Can you work these out from the model? Positions are in its coordinate system, mm. A direction names the side the tool comes from. Round coordinates to 2 decimals unless told otherwise and drop trailing zeros. Write each loop counter-clockwise with the first axis right and the second up, starting at its lowest first coordinate (ties: lowest second). Pieces come first, ordered by that corner, then holes. Notation, with made-up numbers: M -10.5,26 L 48.5,26 A9 cw 48.5,31 Z; hole C 86.25,30.25 d8. An arc over 180 degrees is marked long. Answer as a JSON object with one key per item and string values. Group by question number.
1) Please list where these lines run through material, in increasing order: L1, parallel to X at y = 5.25, z = 2.2; L2, parallel to Z at x = 17.25, y = 7; L3, parallel to Y at x = -2, z = 0.6. Write a range as [from, to].
2) Suppose I cut it at D-D, the plane y = 2.5. Write out the boundary of the cut face in (x, z), and give its area (3 significant figures).
3) Suppose I cut it at C-C, the plane x = 17.25. Write out the boundary of the cut face in (y, z), and give its area (3 significant figures).
4) If we mould it in two halves opening along Y, with no side actions, what happens to faces 5 (the flat face through (10, 3.051, 2)), 6 (the flat face through (7, 8, 0)), 7 (the cylindrical face through (-5.414, 8.228, 0.811)), 8 (the cylindrical face through (-2.325, 7.536, 0.811))? For each: +Y half, -Y half, draft (parallel to the pull), parting line (faces both ways), or undercut.
5) I'm going to push flat-ended pins straight in: pin 1 Ø1.5 at (x, z) = (10, 2.5) entering from -Y; pin 2 Ø1.1 at (y, z) = (6, 2.5) entering from -X; pin 3 Ø0.5 at (y, z) = (2.5, 0.5) entering from +X. Where does each tip first touch, or does it pass through?
6) Suppose I cut it at A-A, the plane z = 0.7. Write out the boundary of the cut face in (x, y).
7) Suppose I cut it at B-B, the plane y = 9. Write out the boundary of the cut face in (x, z).
8) On a 3-axis mill with a long thin cutter (end or side, diameter ignored), from which of +Z, -Z, +X, -X, +Y, -Y can I reach the whole of each face in a straight line? I mean faces 1 (the flat face through (4, 8.379, 2)), 2 (the flat face through (2.571, 7, 2)), 3 (the flat face through (15, 2, 1)), 4 (the flat face through (10, 7.068, 2)). Say none if no direction works.
from build123d import *

# Parameters (mm, degrees)
SKETCH_1_W      = 15
SKETCH_1_H      = 13
EXTRUDE_1_DEPTH = 1.6
SKETCH_2_R      = 3.5
SKETCH_2_R_2    = 1.5
EXTRUDE_2_DEPTH = 1.6
FILLET_1_R      = 2
SKETCH_3_W      = 3.618558991
SKETCH_3_H      = 4.017455257
SKETCH_3_W_2    = 2.3933776
SKETCH_3_H_2    = 3.647051581
EXTRUDE_3_DEPTH = 1.4
EXTRUDE_4_DEPTH = 1.6


with BuildPart() as part:
    # Эскиз1 → Бобышка-Вытянуть1 (new body)
    with BuildSketch(Plane.XY):
        with Locations((7.5, 6.5)):
            Rectangle(SKETCH_1_W, SKETCH_1_H)
    extrude(amount=EXTRUDE_1_DEPTH)

    # Эскиз2 → Бобышка-Вытянуть2 (add)
    # profile 1 of 2: a face of its own
    with BuildSketch(Plane.XY.offset(1.6)):
        with Locations((-2, 9)):
            Circle(SKETCH_2_R)
        with Locations((-2, 9)):
            Circle(SKETCH_2_R_2, mode=Mode.SUBTRACT)
    # profile 2 of 2: a face of its own
    with BuildSketch(Plane.XY.offset(1.6)):
        with Locations((17, 9)):
            Circle(SKETCH_2_R)
        with Locations(Location((17, 9, 0), (0, 0, 180))):
            Circle(SKETCH_2_R_2, mode=Mode.SUBTRACT)
    extrude(amount=-EXTRUDE_2_DEPTH)

    # Скругление1
    fillet_1_edges = [part.edges().sort_by_distance(p)[0] for p in [
        (0, 6.127718677, 0.8),
        (15, 6.127718677, 0.8),
    ]]
    fillet(fillet_1_edges, radius=FILLET_1_R)

    # Эскиз3 → Бобышка-Вытянуть3 (add)
    with BuildSketch(Plane.XY.offset(1.6)):
        with Locations((9.793653534, 5.059744515)):
            Rectangle(SKETCH_3_W, SKETCH_3_H)
        with Locations((3.767470648, 6.555605515)):
            Rectangle(SKETCH_3_W_2, SKETCH_3_H_2)
    extrude(amount=EXTRUDE_3_DEPTH)

    # Эскиз4 → Бобышка-Вытянуть4 (add)
    with BuildSketch(Plane.XY.offset(1.6)):
        with BuildLine():
            Line((-3.62195122, 12.101495485), (7.5, 9.632875059))
            Line((7.5, 9.632875059), (18.62195122, 12.101495485))
            ThreePointArc((18.62195122, 12.101495485), (7.5, 14.834097875), (-3.62195122, 12.101495485))
        make_face()
    extrude(amount=-EXTRUDE_4_DEPTH)


solid = part.part
Results:
{
 "1": {"L1": "[2.57, 4.96], [7.98, 11.6]", "L2": "[0, 1.6]", "L3": "[5.5, 7.5], [10.5, 12.87]"},
 "2": {"outline": "M 0,0 L 15,0 L 15,1.6 L 0,1.6 Z", "area": "24.0 mm^2"},
 "3": {"outline": "M 5.51,0 L 7.52,0 L 7.52,1.6 L 5.51,1.6 Z; M 10.48,0 L 12.76,0 L 12.76,1.6 L 10.48,1.6 Z", "area": "6.88 mm^2"},
 "4": {"face 5": "-Y half", "face 6": "draft", "face 7": "parting line", "face 8": "undercut"},
 "5": {"pin 1": "y = 3.05", "pin 2": "x = 2.57", "pin 3": "x = 15"},
 "6": {"outline": "M -3.62,12.1 A3.5 ccw -2,5.5 A2 cw 0,3.5 L 0,0 L 15,0 L 15,3.5 A2 cw 17,5.5 A3.5 ccw 18.62,12.1 A24 ccw Z; hole C -2,9 d3; hole C 17,9 d3"},
 "7": {"outline": "M -5.5,0 L -3.5,0 L -3.5,1.6 L -5.5,1.6 Z; M -0.5,0 L 15.5,0 L 15.5,1.6 L -0.5,1.6 Z; M 18.5,0 L 20.5,0 L 20.5,1.6 L 18.5,1.6 Z"},
 "8": {"face 1": "+Z, +X, -X, +Y", "face 2": "+Z, -X, +Y, -Y", "face 3": "+Z, -Z, +X, -Y", "face 4": "+Z, +X, +Y"}
}
